Model file for the job. Use its own axes, mm. A direction names the side the tool comes from. Give positions to 0.01 mm unless a question says otherwise; leave off trailing zeros. Loops run counter-clockwise (first coordinate to the right, second up) from the corner with the lowest first, then second, coordinate; pieces in that order, holes last. Notation, with made-up numbers: M 25.25,-17.75 L 63.25,-17.75 A24 cw 63.25,19.25 Z; hole C 69.5,80 d8. An arc over 180 degrees is marked long. Answer in a Markdown table with one row per item.
```python
from build123d import *

# Parameters (mm, degrees)
F0_R     = 25.5
F0_R_2   = 12
F1_DEPTH = 12
F1_TAPER = 5
F2_R     = 30
F2_R_2   = 12
F3_DEPTH = 3
F4_R     = 2
F5_R     = 1


with BuildPart() as f1:
    # F0 (on Top) → F1 (new body)
    with BuildSketch(Plane.XY):
        Circle(F0_R)
        Circle(F0_R_2, mode=Mode.SUBTRACT)
    extrude(amount=F1_DEPTH, taper=F1_TAPER)

    # F2 (on Top) → F3 (join)
    with BuildSketch(Plane.XY):
        Circle(F2_R)
        Circle(F2_R_2, mode=Mode.SUBTRACT)
    extrude(amount=-F3_DEPTH)

    # F4
    f4_edges = [f1.edges().sort_by_distance(p)[0] for p in [
        (-24.450136, 0, 12),
        (-12, 0, -3),
        (-13.049864, 0, 12),
    ]]
    fillet(f4_edges, radius=F4_R)

    # F5
    f5_edges = [f1.edges().sort_by_distance(p)[0] for p in [
        (-30, 0, -3),
        (-30, 0, 0),
    ]]
    fillet(f5_edges, radius=F5_R)


solid = f1.part
```
Q1. Saw through at B-B (z = 6.25). Give the cut face in (x, y), and give its area (3 significant figures).
Reported:
| item | result |
|---|---|
| outline | C 0,0 d49.91; hole C 0,0 d25.09 |
| area | 1,460 mm² |
Q2. Drop flat-ended pins along their axis: pin 1 (5 mm diameter, centred on y = 18.5, z = 5.5, fed in from -X); pin 2 (2 mm diameter, centred on x = -3, z = -1, fed in from -Y); pin 3 (4 mm diameter, centred on x = -13.5, z = 7, fed in from -Y). Give the stop position or say it passes through.
Reported:
| item | result |
|---|---|
| pin 1 | x = -19.25 |
| pin 2 | y = -29.93 |
| pin 3 | y = -22.09 |
Q3. Mould opens along Y. For faces 3 (the face through (15, -5, 12)), 4 (the face through (-9.8, 7.52, 4.03)), 5 (the face through (-11.99, 0.53, -0.49)), 6 (the face through (-19.72, -15.12, 7.42)) say: released by +Y, released by -Y, zero draft, split by the parting line, or undercut.
Reported:
| item | result |
|---|---|
| face 3 | zero draft |
| face 4 | undercut |
| face 5 | undercut |
| face 6 | split by the parting line |
Q4. 3-axis set-ups, long thin cutter, end or side, ignore diameter. For faces 1 (the face through (0, -26, 0)), 2 (the face through (-29.97, 1.32, -1.49)): which of +Z, -Z, +X, -X, +Y, -Y reach the whole face in a straight line?
Reported:
| item | result |
|---|---|
| face 1 | +Z |
| face 2 | +Z, -Z |
Q5. Saw through at A-A (x = 0). Give the cut face in (y, z).
Reported:
| item | result |
|---|---|
| outline | M -30,-2 A1 ccw -29,-3 L -14,-3 A2 ccw -12,-1 L -12,0 L -12.89,10.17 A2 ccw -14.88,12 L -22.62,12 A2 ccw -24.61,10.17 L -25.5,0 L -29,0 A1 ccw -30,-1 Z; M 12,-1 A2 ccw 14,-3 L 29,-3 A1 ccw 30,-2 L 30,-1 A1 ccw 29,0 L 25.5,0 L 24.61,10.17 A2 ccw 22.62,12 L 14.88,12 A2 ccw 12.89,10.17 L 12,0 Z |
Q6. Probe probe 1 along Z at (x, y) = (11, 24.5); probe 2 along Y at (x, z) = (0, -0.2); probe 3 along X at (y, z) = (-3, 1). List the from-to ranges inside material, lowest first.
Reported:
| item | result |
|---|---|
| probe 1 | -3 to 0 |
| probe 2 | -29.6 to -12, 12 to 29.6 |
| probe 3 | -25.23 to -11.71, 11.71 to 25.23 |
